from build123d import *

# Parameters (mm, degrees)
PAD_DEPTH    = 25
PAD001_DEPTH = 10
FILLET_R     = 12.5
FILLET001_R  = 12.5
FILLET002_R  = 5
FILLET003_R  = 5
SKETCH002_R  = 5
POCKET_DEPTH = 10.001


with BuildPart() as part:
    # Sketch → Pad (new body, symmetric)
    with BuildSketch(Plane.XZ):
        with BuildLine():
            Line((-50, 0), (-20, 0))
            ThreePointArc((20, 0), (0, 20), (-20, 0))
            Line((20, 0), (50, 0))
            Line((50, 0), (50, 10))
            Line((28.284271, 10), (50, 10))
            ThreePointArc((28.284271, 10), (0, 30), (-28.284271, 10))
            Line((-50, 10), (-28.284271, 10))
            Line((-50, 0), (-50, 10))
        make_face()
    extrude(amount=PAD_DEPTH, both=True)

    # Sketch001 → Pad001 (new body)
    with BuildSketch(Plane(origin=(50, 0, 0), x_dir=(0, 0, 1), z_dir=(1, 0, 0))):
        with BuildLine():
            Line((0, 25), (40, 25))
            Line((40, 25), (40, 7.5))
            Line((40, 7.5), (24.999965, 7.5))
            ThreePointArc((24.999965, 7.5), (17.5, -1.8e-05), (25, -7.5))
            Line((40, -7.5), (25, -7.5))
            Line((40, -25), (40, -7.5))
            Line((0, -25), (40, -25))
            Line((0, 25), (0, -25))
        make_face()
    extrude(amount=-PAD001_DEPTH)

    # Fillet
    fillet_edges = [part.edges().sort_by_distance(p)[0] for p in [
        (-50, -25, 5),
    ]]
    fillet(fillet_edges, radius=FILLET_R)

    # Fillet001
    fillet001_edges = [part.edges().sort_by_distance(p)[0] for p in [
        (-50, 25, 5),
    ]]
    fillet(fillet001_edges, radius=FILLET001_R)

    # Fillet002
    fillet002_edges = [part.edges().sort_by_distance(p)[0] for p in [
        (45, -25, 40),
    ]]
    fillet(fillet002_edges, radius=FILLET002_R)

    # Fillet003
    fillet003_edges = [part.edges().sort_by_distance(p)[0] for p in [
        (45, 25, 40),
    ]]
    fillet(fillet003_edges, radius=FILLET003_R)

    # Sketch002 → Pocket (cut, through all)
    with BuildSketch(Plane(origin=(0, 0, 10), x_dir=(-1, 0, 0), z_dir=(0, 0, 1))):
        with Locations((37.5, 12.5)):
            Circle(SKETCH002_R)
        with Locations((37.5, -12.5)):
            Circle(SKETCH002_R)
    extrude(amount=-POCKET_DEPTH, mode=Mode.SUBTRACT)


solid = part.part
Geometry: final body of the model. Coordinates: model frame, mm. A direction names the side the tool comes from. Give positions to 0.01 mm unless a question says otherwise; leave off trailing zeros. Order: outer loops, then holes, each group sorted by start corner. A loop starts at its lowest first (then second) coordinate and runs counter-clockwise, first axis right, second up. Notation, with made-up numbers: (55.5, 67.5) -> (59.5, 67.5) arc R5 cw to (59.5, 71.5) -> close; hole circle Ø1 at (-16.5, 39.25). An arc over 180 degrees is marked (long way). Write each question's results on one line, items separated by ' | '.
1) First-contact query: pin 1 Ø24 at (x, y) = (-37, -12) entering from +Z; pin 2 Ø5 at (y, z) = (11, 16.5) entering from -X; pin 3 Ø24 at (y, z) = (11, 22.5) entering from -X. Flat tips, straight axial feed; report the tip coordinate or a pass-through.
Geometry says:
pin 1: stops at z = 16.58 | pin 2: stops at x = -26.53 | pin 3: stops at x = -28.1
2) Cut plane C-C (z = 6). Output: boundary loops of the cut face in (x, y).
Geometry says:
outline: (-50, -12.5) arc R12.5 ccw to (-37.5, -25) -> (-19.08, -25) -> (-19.08, 25) -> (-37.5, 25) arc R12.5 ccw to (-50, 12.5) -> close; (19.08, -25) -> (50, -25) -> (50, 25) -> (19.08, 25) -> close; hole circle Ø10 at (-37.5, -12.5); hole circle Ø10 at (-37.5, 12.5)
3) Draft query along X for faces 4 (the face through (-32.505, -12.72, 5.07)), 5 (the face through (-32.505, 12.28, 5.07)), 6 (the face through (45, -7.5, 33)), 7 (the face through (-50, 0, 5)). Return one class per face: released by +X, released by -X, zero draft, split by the parting line, or undercut.
Geometry says:
face 4: undercut | face 5: undercut | face 6: zero draft | face 7: released by -X
4) Line query: line 1 along Y through (x, z) = (-37.5, 4.25); line 2 along X through (y, z) = (-12, 3); line 3 along Z through (x, y) = (33.5, -11). Output: solid intervals per line, ascending.
Geometry says:
line 1: y = -25 to -17.5, -7.5 to 7.5, 17.5 to 25 | line 2: x = -50 to -42.47, -32.53 to -19.77, 19.77 to 50 | line 3: z = 0 to 10
5) Set-up query: faces 1 (the face through (-39, 0, 10)), 2 (the face through (34, 0, 10)), 3 (the face through (45, 7.5, 33)). Return all of +Z, -Z, +X, -X, +Y, -Y with unobstructed straight access to the full face (end or side cutting, diameter ignored); none if empty.
Geometry says:
face 1: +Z, -X, +Y, -Y | face 2: +Z, +Y, -Y | face 3: +Z, +X
6) Cut plane B-B (y = 9). Output: boundary loops of the cut face in (x, z), and give its area (3 significant figures).
Geometry says:
outline: (-50, 0) -> (-41.07, 0) -> (-41.07, 10) -> (-50, 10) -> close; (-33.93, 0) -> (-20, 0) arc R20 cw to (20, 0) -> (50, 0) -> (50, 40) -> (40, 40) -> (40, 10) -> (28.28, 10) arc R30 ccw to (-28.28, 10) -> (-33.93, 10) -> close | area: 1,430 mm²
7) Cut plane D-D (x = -39). Output: boundary loops of the cut face in (y, z), and give its area (3 significant figures).
Geometry says:
outline: (-24.91, 0) -> (-17.27, 0) -> (-17.27, 10) -> (-24.91, 10) -> close; (-7.73, 0) -> (7.73, 0) -> (7.73, 10) -> (-7.73, 10) -> close; (17.27, 0) -> (24.91, 0) -> (24.91, 10) -> (17.27, 10) -> close | area: 307 mm²
8) Cut plane A-A (z = 33.5). Output: boundary loops of the cut face in (x, y), and give its area (3 significant figures).
Geometry says:
outline: (40, -25) -> (50, -25) -> (50, -7.5) -> (40, -7.5) -> close; (40, 7.5) -> (50, 7.5) -> (50, 25) -> (40, 25) -> close | area: 350 mm²
